Could you check a few things on this model? Use its own coordinates, in mm. Face numbers are marked on the shaded views. A direction names the side the tool comes from. Round coordinates to 2 decimals unless told otherwise and drop trailing zeros. Loops run counter-clockwise (first coordinate to the right, second up) from the corner with the lowest first, then second, coordinate; pieces in that order, holes last. Notation, with made-up numbers: (2.25, -24) - (44.25, -24) arc R31 ccw to (44.25, 9) - close; hole circle Ø5 at (-6.75, 29.25). An arc over 180 degrees is marked (long way). Use one line per item in the form item = value.
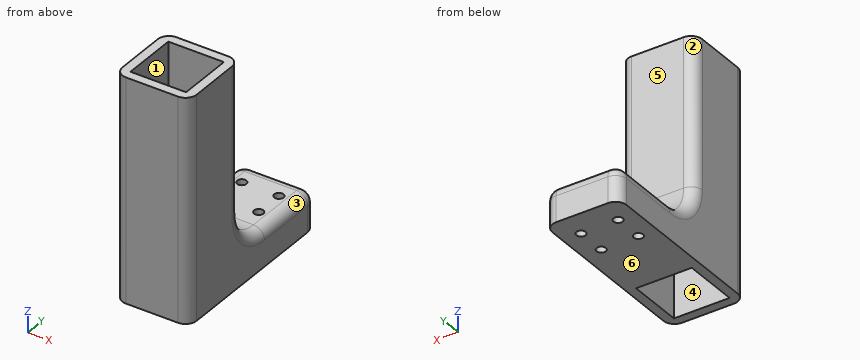
```python
from build123d import *

# Parameters (mm, degrees)
SKETCH_4_W      = 20
SKETCH_4_H      = 20
SKETCH_4_W_2    = 15
SKETCH_4_H_2    = 15
EXTRUDE_3_DEPTH = 60
SKETCH_5_W      = 20
SKETCH_5_H      = 30
EXTRUDE_4_DEPTH = 10
M3X0_5_1_D      = 2.5
FILLET_1_R      = 10
FILLET_2_R      = 3
FILLET_3_R      = 3


with BuildPart() as part:
    # ｽｹｯﾁ4 → ﾎﾞｽ - 押し出し3 (new body)
    with BuildSketch(Plane.XY):
        Rectangle(SKETCH_4_W, SKETCH_4_H)
        Rectangle(SKETCH_4_W_2, SKETCH_4_H_2, mode=Mode.SUBTRACT)
    extrude(amount=EXTRUDE_3_DEPTH)

    # ｽｹｯﾁ5 → ﾎﾞｽ - 押し出し4 (add)
    with BuildSketch(Plane.XY):
        with Locations((0, 25)):
            Rectangle(SKETCH_5_W, SKETCH_5_H)
    extrude(amount=EXTRUDE_4_DEPTH)

    # M3x0.5 ねじ穴1 (through all)
    with Locations(Plane(origin=(0, 0, 0), x_dir=(-1, 0, 0), z_dir=(0, 0, -1))):
        with Locations((-5, 25), (-5, 33), (5, 33), (5, 25)):
            Hole(M3X0_5_1_D / 2)

    # ﾌｨﾚｯﾄ1
    fillet_1_edges = [part.edges().sort_by_distance(p)[0] for p in [
        (0, 10, 10),
    ]]
    fillet(fillet_1_edges, radius=FILLET_1_R)

    # ﾌｨﾚｯﾄ2
    fillet_2_edges = [part.edges().sort_by_distance(p)[0] for p in [
        (10, 40, 5),
        (-10, 40, 5),
        (0, 40, 10),
        (-10, 30, 10),
        (10, 30, 10),
        (10, 12.928932188, 12.928932188),
        (-10, 12.928932188, 12.928932188),
        (-10, 10, 40),
        (10, 10, 40),
    ]]
    fillet(fillet_2_edges, radius=FILLET_2_R)

    # ﾌｨﾚｯﾄ3
    fillet_3_edges = [part.edges().sort_by_distance(p)[0] for p in [
        (10, -10, 30),
        (-10, -10, 30),
    ]]
    fillet(fillet_3_edges, radius=FILLET_3_R)


solid = part.part
```
1. For P1, Ø4, axis at x = -0.5, y = 27, coming from the +Z side; P2, Ø3, axis at x = 5, z = 17.5, coming from the +Y side; P3, Ø4.5, axis at x = -3.5, z = 15.5, coming from the +Y side, each with a flat end and sliding along its axis, tell me the tip position at first contact or that it passes through.
Solution:
P1 = 10
P2 = 10.83
P3 = 12.62
2. If we section it at C-C, the plane z = 5.5: Write out the boundary of the cut face in (x, y), plus the area to 3 significant figures.
Solution:
outline = (-10, -7) arc R3 ccw to (-7, -10) - (7, -10) arc R3 ccw to (10, -7) - (10, 37) arc R3 ccw to (7, 40) - (-7, 40) arc R3 ccw to (-10, 37) - close; hole (-7.5, -7.5) - (7.5, -7.5) - (7.5, 7.5) - (-7.5, 7.5) - close; hole circle Ø2.5 at (-5, 25); hole circle Ø2.5 at (-5, 33); hole circle Ø2.5 at (5, 25); hole circle Ø2.5 at (5, 33)
area = 748 mm^2
3. On a 3-axis mill with a long thin cutter (end or side, diameter ignored), from which of +Z, -Z, +X, -X, +Y, -Y can I reach the whole of each face in a straight line? I mean the marked faces 1, 2 and 3. Say none if no direction works.
Solution:
face_1 = +Z, -Z
face_2 = +Z, -X, +Y
face_3 = +Z, +X, +Y
4. If we section it at A-A, the plane x = -5: Write out the boundary of the cut face in (y, z), plus the area to 3 significant figures.
Solution:
outline = (-10, 0) - (-7.5, 0) - (-7.5, 60) - (-10, 60) - close; (7.5, 0) - (23.75, 0) - (23.75, 10) - (20, 10) arc R10 cw to (10, 20) - (10, 60) - (7.5, 60) - close; (26.25, 0) - (31.75, 0) - (31.75, 10) - (26.25, 10) - close; (34.25, 0) - (40, 0) - (40, 7) arc R3 ccw to (37, 10) - (34.25, 10) - close
area = 570 mm^2
5. We'd pull the mould along Y, two halves only. Please class the marked faces 4, 5 and 6: +Y half, -Y half, draft (parallel to the pull), parting line (faces both ways), or undercut.
Solution:
face_4 = undercut
face_5 = +Y half
face_6 = draft
6. If we section it at D-D, the plane y = 33: Write out the boundary of the cut face in (x, z), plus the area to 3 significant figures.
Solution:
outline = (-10, 0) - (-6.25, 0) - (-6.25, 10) - (-7, 10) arc R3 ccw to (-10, 7) - close; (-3.75, 0) - (3.75, 0) - (3.75, 10) - (-3.75, 10) - close; (6.25, 0) - (10, 0) - (10, 7) arc R3 ccw to (7, 10) - (6.25, 10) - close
area = 146 mm^2
7. Please list where these lines run through material, in increasing order: line 1 along Y through (x, z) = (5, 5.5); line 2 along X through (y, z) = (-7, 4).
Solution:
line_1 = -10 to -7.5, 7.5 to 23.75, 26.25 to 31.75, 34.25 to 40
line_2 = -10 to -7.5, 7.5 to 10
8. If we section it at B-B, the plane y = -4.5: Write out the boundary of the cut face in (x, z).
Solution:
outline = (-10, 0) - (-7.5, 0) - (-7.5, 60) - (-10, 60) - close; (7.5, 0) - (10, 0) - (10, 60) - (7.5, 60) - close
